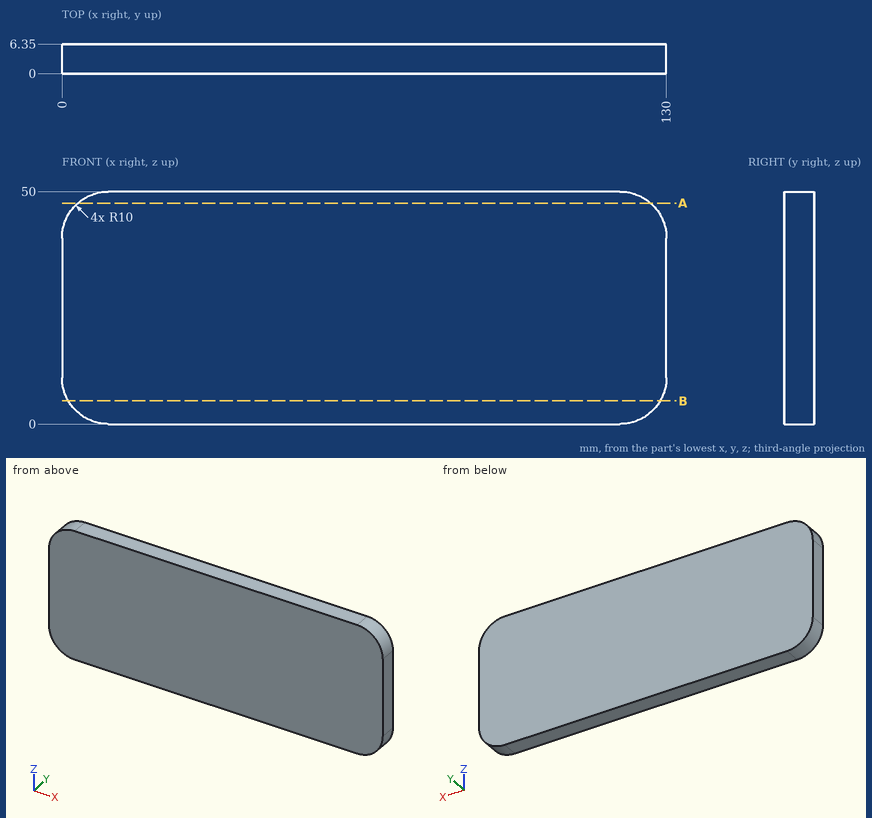
Geometry: see drawing. Coordinates: mm, zero at the bounding-box minimum. Give positions to 0.01 mm unless a question says otherwise; leave off trailing zeros. Order: outer loops, then holes, each group sorted by start corner. A loop starts at its lowest first (then second) coordinate and runs counter-clockwise, first axis right, second up. Notation, with made-up numbers: (12, 33) - (64, 33) arc R22 ccw to (64, 49) - close; hole circle Ø1 at (-38.5, 25). An arc over 180 degrees is marked (long way). Use CSV: the item, a comma, the result in double quotes.
1. Section query A-A (z = 47.5). Output: boundary loops of the cut face in (x, y).
Answers below:
outline,"(3.39, 0) - (126.61, 0) - (126.61, 6.35) - (3.39, 6.35) - close"
2. Section query B-B (z = 5). Output: boundary loops of the cut face in (x, y), plus the area to 3 significant figures.
Answers below:
outline,"(1.34, 0) - (128.66, 0) - (128.66, 6.35) - (1.34, 6.35) - close"
area,"808 mm2"
3. Material intervals for line 1 along X through (y, z) = (4.75, 6); line 2 along X through (y, z) = (6, 45.5), sorted ascending. Write a range as from..to.
Answers below:
line 1,"0.83..129.17"
line 2,"1.65..128.35"
